The model under review builds one solid part; all positions refer to its coordinate system, in mm. Face numbers are marked on the shaded views. A direction names the side the tool comes from. Give positions to 0.01 mm unless a question says otherwise; leave off trailing zeros. Write item = value, one per line. Start each with the question number.
1. Wall thickness on probe 1 along Y at (x, z) = (-15.5, 5.75); probe 2 along X at (y, z) = (0.5, 4); probe 3 along X at (y, z) = (-7.5, 1): over which ranges is each line inside the solid? List them lowest first.
2. Mouldability with a two-part tool opening along Y and no side actions: class the marked faces 4, 5 and 6 as pulls with the +Y half, pulls with the -Y half, needs draft (parallel to the pull), parting line crosses it, or undercut.
3. Machinability: for the marked faces 1, 2 and 3, which of the approach directions +Z, -Z, +X, -X, +Y, -Y give a long, thin tool a straight path to every point of the face, cutting with its end or side? Answer none if there is none.
4. We need section A-A, the plane x = 0. State how many separate pieces and enclosed holes the cut face has, and give its area (3 significant figures).
5. For P1, Ø1, axis at x = -13.5, z = 9.5, coming from the +Y side; P2, Ø5, axis at y = 0.5, z = -5, coming from the +X side; P3, Ø6, axis at x = 15.5, z = 4.5, coming from the -Y side, all flat-tipped, find the tip position at first contact; note any pin that passes through.
from build123d import *

# Parameters (mm, degrees)
CUT_EXTRUDE1_REACH = 48.701
CIRPATTERN1_COUNT  = 8
CHAMFER1_SIZE      = 2.54
CUT_EXTRUDE2_REACH = 43.904
SKETCH3_R          = 2.5


with BuildPart() as part:
    # Sketch1 → Revolve1 (revolve)
    with BuildSketch(Plane(origin=(0, 0, 0), x_dir=(0, 0, -1), z_dir=(1, 0, 0)), mode=Mode.PRIVATE) as revolve1_sk:
        Polygon((-6.61, 0), (1.61, 0), (1.61, 2.6), (1.61, 5.5), (-7.28, 22.352), (9.23, 22.352), (9.23, 27.432), (6.69, 27.432), (6.69, 26), (-14.23, 26), (-14.23, 27.432), (-16.77, 27.432), (-16.77, 22.352), (-6.61, 5.5), align=None)
    revolve(revolve1_sk.sketch.rotate(Axis((0, 0, 6.61), (0, 0, -1)), 180), axis=Axis((0, 0, 6.61), (0, 0, -1)))

    # Cut-Extrude1: up to this cone (the profile starts inside it)
    cut_extrude1_end = Plane(origin=(0, 0, 16.77), z_dir=(0, 0, 1)).offset(-21.281435031) * Cone(1.896e-06, 210.079048668, 110.82380286, align=(Align.CENTER, Align.CENTER, Align.MIN), mode=Mode.PRIVATE)
    # Sketch2 → Cut-Extrude1 (cut, up to the surface)
    with BuildSketch(Plane.XY.offset(16.77), mode=Mode.PRIVATE) as cut_extrude1_sk1:
        with BuildLine():
            Line((-5.259202996, 19.62761279), (-1.643500936, 6.133628997))
            ThreePointArc((-1.643500936, 6.133628997), (0, 6.35), (1.643500936, 6.133628997))
            Line((1.643500936, 6.133628997), (5.259202996, 19.62761279))
            ThreePointArc((5.259202996, 19.62761279), (0, 20.32), (-5.259202996, 19.62761279))
        make_face()
    cut_extrude1_tool1 = extrude(cut_extrude1_sk1.sketch, amount=-CUT_EXTRUDE1_REACH, mode=Mode.PRIVATE) & cut_extrude1_end
    cut_extrude1 = cut_extrude1_tool1.solids().sort_by_distance((0, 14.388913, 16.77))[0]
    add(cut_extrude1, mode=Mode.SUBTRACT)

    # CirPattern1: Cut-Extrude1 ×8 about axis
    cirpattern1_axis = Axis((0, 0, 0), (0, 0, 1))
    for i in range(1, CIRPATTERN1_COUNT):
        add(cut_extrude1.rotate(cirpattern1_axis, i * 360 / CIRPATTERN1_COUNT), mode=Mode.SUBTRACT)

    # Chamfer1
    chamfer1_edges = [part.edges().sort_by_distance(p)[0] for p in [
        (0, 22.352, -9.23),
    ]]
    chamfer(chamfer1_edges, length=CHAMFER1_SIZE)

    # Sketch3 → Cut-Extrude2 (cut, up to next)
    with BuildSketch(Plane.XY.offset(6.61), mode=Mode.PRIVATE) as cut_extrude2_sk1:
        Circle(SKETCH3_R)
    cut_extrude2_tool1 = extrude(cut_extrude2_sk1.sketch, amount=-CUT_EXTRUDE2_REACH, mode=Mode.PRIVATE) & part.part
    add(cut_extrude2_tool1.solids().sort_by_distance((0, 0, 6.61))[0], mode=Mode.SUBTRACT)


solid = part.part
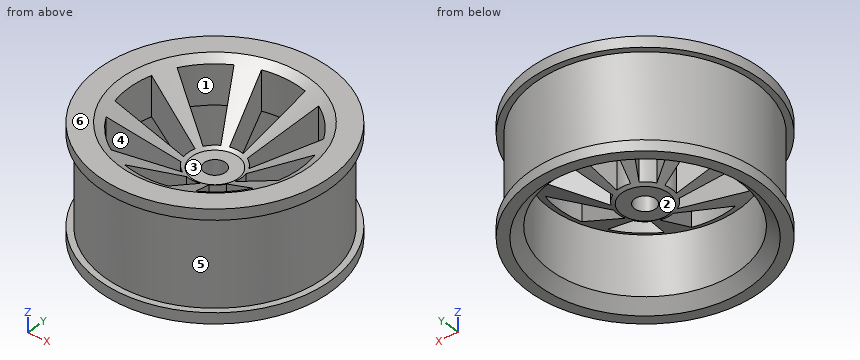
Model answer:
q1.probe_1 = -20.87 to -16.1, -8.95 to -4.15, 4.15 to 8.95, 16.1 to 20.87
q1.probe_2 = -26 to -22.35, -6.33 to -2.45, 2.45 to 6.33, 22.35 to 26
q1.probe_3 = -24.89 to -21.06, -4.33 to -2.01, 2.01 to 4.33, 21.06 to 24.89
q2.face_4 = undercut
q2.face_5 = parting line crosses it
q2.face_6 = needs draft
q3.face_1 = +Z, -Z
q3.face_2 = -Z
q3.face_3 = +Z
q4.separate_pieces = 4
q4.enclosed_holes = 0
q4.area = 299 mm2
q5.P1 = 22.52
q5.P2 = 27.43
q5.P3 = -22.8
